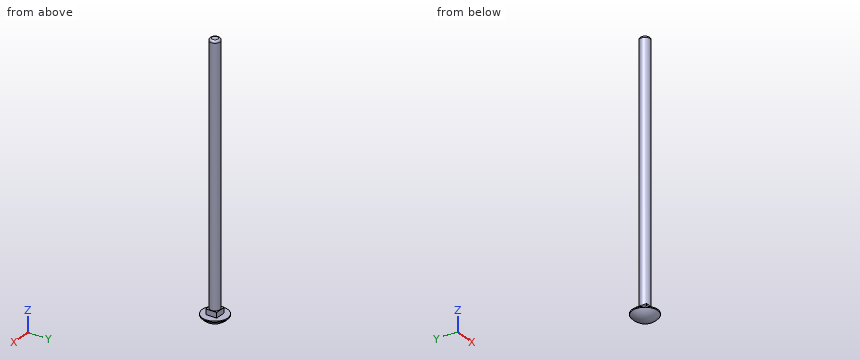
```python
from build123d import *

# Parameters (mm, degrees)
F0_R     = 3.048
F1_DEPTH = 152.4
F2_W     = 6.5278
F2_H     = 6.5278
F3_DEPTH = 3.175
F4_R     = 7.6835
F5_DEPTH = 0.635
F8_R     = 1.27


with BuildPart() as f1:
    # F0 (on Top) → F1 (new body)
    with BuildSketch(Plane.XY):
        Circle(F0_R)
    extrude(amount=F1_DEPTH)

    # F2 (on Top) → F3 (join)
    with BuildSketch(Plane.XY):
        Rectangle(F2_W, F2_H)
    extrude(amount=-F3_DEPTH)

    # F4 (on face) → F5 (join)
    with BuildSketch(Plane(origin=(0, 0, -3.175), x_dir=(1, 0, 0), z_dir=(0, 0, -1))):
        Circle(F4_R)
    extrude(amount=F5_DEPTH)

    # F6 (on Front) → F7 (revolve)
    with BuildSketch(Plane.XZ):
        with BuildLine():
            Line((0, -3.81), (0, -7.62))
            ThreePointArc((0, -7.62), (4.288131, -6.615202), (7.6835, -3.81))
            Line((7.6835, -3.81), (0, -3.81))
        make_face()
    revolve(axis=Axis((0, 0, -5.715), (0, 0, -1)))

    # F8
    f8_edges = [f1.edges().sort_by_distance(p)[0] for p in [
        (-3.048, 0, 152.4),
    ]]
    fillet(f8_edges, radius=F8_R)


solid = f1.part
```
Check sheet for the modelled part. Datum: model origin and axes. Units: mm. Give positions to 0.01 mm unless a question says otherwise; leave off trailing zeros. Loops run counter-clockwise (first coordinate to the right, second up) from the corner with the lowest first, then second, coordinate; pieces in that order, holes last. Notation, with made-up numbers: (49, 86.25) - (83, 86.25) arc R19 ccw to (83, 123.25) - close; hole circle Ø10 at (2.25, 21). An arc over 180 degrees is marked (long way). One line per question, with ' | ' between items. Start each with the question number.
1. Gauge pin test, flat ends, axial feed: pin 1 Ø1.6 at (x, z) = (1, -1.5) entering from +Y; pin 2 Ø4 at (y, z) = (2, 68.5) entering from -X; pin 3 Ø3 at (y, z) = (2.5, 88) entering from +X. Record the tip position at first contact, or that the pin passes through.
2. Material ranges on line 1 along X through (y, z) = (-1.25, 64.5); line 2 along X through (y, z) = (-1.75, 143); line 3 along Z through (x, y) = (4, -2.25) (3 decimals), recorded low to high. Write a range as [from, to].
3. Cross-section at A-A, the plane z = 127. Enter the section's corners in (x, y), plus the area to 3 significant figures.
Check result:
1) pin 1: stops at y = 3.26 | pin 2: stops at x = -3.05 | pin 3: stops at x = 2.88
2) line 1: x = [-2.78, 2.78] | line 2: x = [-2.5, 2.5] | line 3: z = [-6.459, -3.175]
3) outline: circle Ø6.1 at (0, 0) | area: 29.2 mm2
